Could you check a few things on this model? Use its own coordinates, in mm. A direction names the side the tool comes from. Coordinates: 2 decimals unless noted, no trailing zeros. Write each loop counter-clockwise with the first axis right and the second up, starting at its lowest first coordinate (ties: lowest second). Pieces come first, ordered by that corner, then holes.
```python
from build123d import *

# Parameters (mm, degrees)
BOSS_EXTRUDE1_REACH        = 91.067
BOSS_EXTRUDE1_START_RADIUS = 14.5
BOSS_EXTRUDE1_END_RADIUS   = 14.5
SKETCH5_W                  = 8
SKETCH5_H                  = 10
CUT_EXTRUDE1_START         = -10
CUT_EXTRUDE1_DEPTH         = 10
SKETCH8_R                  = 1.75
CUT_EXTRUDE2_DEPTH         = 3
CUT_EXTRUDE3_START         = -3
SKETCH9_R                  = 1.75
CUT_EXTRUDE3_DEPTH         = 3
CUT_EXTRUDE5_DEPTH         = 10
CUT_EXTRUDE8_START         = -10
CUT_EXTRUDE8_DEPTH         = 10
SKETCH13_R                 = 0.6
CUT_EXTRUDE9_DEPTH         = 3


# Read off the part's stored shape, not the designer's step: Cut-Extrude1, Cut-Extrude8
with BuildPart() as part:
    # Sketch1 → Revolve1 (revolve)
    with BuildSketch(Plane.XY, mode=Mode.PRIVATE) as revolve1_sk:
        with BuildLine():
            Line((12, 0), (14.5, 0))
            Line((14.5, 0), (14.5, 80))
            ThreePointArc((14.5, 80), (13.849763488, 82.244753612), (12.100400466, 83.794416583))
            Line((12.100400466, 83.794416583), (8.5, 83.794416583))
            Line((8.5, 83.794416583), (8.5, 80))
            Line((8.5, 80), (12, 80))
            Line((12, 80), (12, 0))
        make_face()
    revolve(revolve1_sk.sketch.rotate(Axis((0, 0, 0), (0, 1, 0)), 90), axis=Axis((0, 0, 0), (0, 1, 0)))

    # Boss-Extrude1: from a cylinder face, 91.067 long prism both ways, kept between that surface and its translate by the depth
    boss_extrude1_start = Plane(origin=(0, 24.058844, 0), z_dir=(0, -1, 0)) * Cylinder(BOSS_EXTRUDE1_START_RADIUS, 249.016312, mode=Mode.PRIVATE)
    boss_extrude1_end = Plane(origin=(2.8, 24.058844, 0), z_dir=(0, -1, 0)) * Cylinder(BOSS_EXTRUDE1_END_RADIUS, 249.016312, mode=Mode.PRIVATE)
    # Sketch5 → Boss-Extrude1 (add, from a surface)
    with BuildSketch(Plane(origin=(0, 0, 0), x_dir=(0, 0, -1), z_dir=(1, 0, 0)), mode=Mode.PRIVATE) as boss_extrude1_sk1:
        with Locations((-0.003167699, 5.61768818)):
            Rectangle(SKETCH5_W, SKETCH5_H)
    boss_extrude1_tool1 = extrude(boss_extrude1_sk1.sketch, amount=BOSS_EXTRUDE1_REACH, both=True, mode=Mode.PRIVATE)
    # Sketch5 → Boss-Extrude1 (add, from a surface)
    with BuildSketch(Plane(origin=(0, 0, 0), x_dir=(0, 0, -1), z_dir=(1, 0, 0)), mode=Mode.PRIVATE) as boss_extrude1_sk2:
        with Locations((0, 42.5)):
            Rectangle(SKETCH5_W, SKETCH5_H)
    boss_extrude1_tool2 = extrude(boss_extrude1_sk2.sketch, amount=BOSS_EXTRUDE1_REACH, both=True, mode=Mode.PRIVATE)
    boss_extrude1 = ((boss_extrude1_tool1 - boss_extrude1_start) & boss_extrude1_end).solids().sort_by_distance((15.337359, 5.617688, 0.003168))[0] + ((boss_extrude1_tool2 - boss_extrude1_start) & boss_extrude1_end).solids().sort_by_distance((15.337359, 5.617688, 0.003168))[0]
    add(boss_extrude1)

    # Cut-Extrude1 outline → Cut-Extrude1 (cut)
    with BuildSketch(Plane(origin=(0, 47.5, 0), x_dir=(1, 0, 0), z_dir=(0, 1, 0)).offset(CUT_EXTRUDE1_START)):
        with BuildLine():
            Line((16.737359865, 4), (13.937359865, 4))
            Line((13.937359865, 4), (16.863384202, 3.531462132))
            ThreePointArc((16.863384202, 3.531462132), (16.802331913, 3.766258222), (16.737359865, 4))
        make_face()
        with BuildLine():
            ThreePointArc((16.737359865, -4), (16.802331913, -3.766258222), (16.863384202, -3.531462132))
            Line((16.863384202, -3.531462132), (13.937359865, -4))
            Line((13.937359865, -4), (16.737359865, -4))
        make_face()
        with BuildLine():
            ThreePointArc((16.863384202, -3.531462132), (17.3, 0), (16.863384202, 3.531462132))
            Line((16.863384202, 3.531462132), (16.863384202, -3.531462132))
        make_face()
    cut_extrude1 = extrude(amount=CUT_EXTRUDE1_DEPTH, mode=Mode.SUBTRACT)

    # Mirror2: Boss-Extrude1, Cut-Extrude1 across plane
    add(boss_extrude1.mirror(Plane(origin=(0, 0, 0), x_dir=(0, 0, 1), z_dir=(1, 0, 0))))
    add(cut_extrude1.mirror(Plane(origin=(0, 0, 0), x_dir=(0, 0, 1), z_dir=(1, 0, 0))), mode=Mode.SUBTRACT)

    # Sketch8 → Cut-Extrude2 (cut)
    with BuildSketch(Plane.ZY.offset(16.863384202)):
        with Locations((0.02126458, 42.512867657)):
            Circle(SKETCH8_R)
    extrude(amount=-CUT_EXTRUDE2_DEPTH, mode=Mode.SUBTRACT)

    # Sketch9 → Cut-Extrude3 (cut)
    with BuildSketch(Plane(origin=(16.863384202, 0, 0), x_dir=(0, 0, -1), z_dir=(1, 0, 0)).offset(CUT_EXTRUDE3_START)):
        with Locations(Location((-0.02126458, 42.512867657, 0), (0, 0, 180))):
            Circle(SKETCH9_R)
    extrude(amount=CUT_EXTRUDE3_DEPTH, mode=Mode.SUBTRACT)

    # Sketch11 → Cut-Extrude5 (cut)
    with BuildSketch(Plane(origin=(0, 10.61768818, 0), x_dir=(1, 0, 0), z_dir=(0, 1, 0))):
        with BuildLine():
            Line((-13.9382686, 3.996832301), (-16.7382686, 3.996832301))
            ThreePointArc((-16.7382686, 3.996832301), (-17.299999625, -0.003295577), (-16.73645035, -4.003167699))
            Line((-16.73645035, -4.003167699), (-13.93645035, -4.003167699))
            ThreePointArc((-13.93645035, -4.003167699), (-14.499999625, -0.003295577), (-13.9382686, 3.996832301))
        make_face()
    extrude(amount=-CUT_EXTRUDE5_DEPTH, mode=Mode.SUBTRACT)

    # Cut-Extrude8 outline → Cut-Extrude8 (cut)
    with BuildSketch(Plane(origin=(0, 10.61768818, 0), x_dir=(1, 0, 0), z_dir=(0, 1, 0)).offset(CUT_EXTRUDE8_START)):
        with BuildLine():
            Line((16.7382686, 3.996832301), (13.9382686, 3.996832301))
            Line((13.9382686, 3.996832301), (17.052533954, 2.667447447))
            ThreePointArc((17.052533954, 2.667447447), (16.91106492, 3.335842745), (16.7382686, 3.996832301))
        make_face()
        with BuildLine():
            ThreePointArc((16.73645035, -4.003167699), (16.910306381, -3.339049838), (17.052533954, -2.667447447))
            Line((17.052533954, -2.667447447), (13.93645035, -4.003167699))
            Line((13.93645035, -4.003167699), (16.73645035, -4.003167699))
        make_face()
        with BuildLine():
            ThreePointArc((17.052533954, -2.667447447), (17.3, 0), (17.052533954, 2.667447447))
            Line((17.052533954, 2.667447447), (17.052533954, -2.667447447))
        make_face()
    extrude(amount=CUT_EXTRUDE8_DEPTH, mode=Mode.SUBTRACT)

    # Sketch13 → Cut-Extrude9 (cut)
    with BuildSketch(Plane(origin=(17.052533954, 0, 0), x_dir=(0, 0, -1), z_dir=(1, 0, 0))):
        with Locations((0, 4.61768818)):
            Circle(SKETCH13_R)
    extrude(amount=-CUT_EXTRUDE9_DEPTH, mode=Mode.SUBTRACT)


solid = part.part
```
1. Please list where these lines run through material, in increasing order: line 1 along X through (y, z) = (59, 0); line 2 along X through (y, z) = (7.5, -7.75); line 3 along Z through (x, y) = (0.5, 59.5).
Verdict:
line 1: x = -14.5 to -12, 12 to 14.5
line 2: x = -12.26 to -9.16, 9.16 to 12.26
line 3: z = -14.49 to -11.99, 11.99 to 14.49
2. On a 3-axis mill with a long thin cutter (end or side, diameter ignored), from which of +Z, -Z, +X, -X, +Y, -Y can I reach the whole of each face in a straight line? I mean faces 4 (the face through (13.863, 42, 0)), 5 (the face through (15.474, 5.548, -3.341)), 6 (the face through (-15.384, 44.248, -0.207)). Say none if no direction works.
Verdict:
face 4: +X
face 5: -Z, +X, -Y
face 6: -X
3. I want a section at A-A on x = 0. Please give me the cut outline in (y, z), plus the area to 3 significant figures.
Verdict:
outline: (0, -14.5) - (80, -14.5) arc R4.2 ccw to (83.79, -12.1) - (83.79, -8.5) - (80, -8.5) - (80, -12) - (0, -12) - close; (0, 12) - (80, 12) - (80, 8.5) - (83.79, 8.5) - (83.79, 12.1) arc R4.2 ccw to (80, 14.5) - (0, 14.5) - close
area: 440 mm2
4. If we mould it in two halves opening along Y, with no side actions, what happens to faces 1 (the face through (-13.863, 43, 0)), 2 (the face through (-8.2, 80, -2.8)), 3 (the face through (-16.863, 41, 2))? For each: pulls with the +Y half, pulls with the -Y half, needs draft (parallel to the pull), parting line crosses it, or undercut.
Verdict:
face 1: undercut
face 2: pulls with the -Y half
face 3: needs draft
5. I want a section at B-B on y = 61. Please give me the cut outline in (x, z).
Verdict:
outline: circle Ø29 at (0, 0); hole circle Ø24 at (0, 0)
6. For pin 1 (2.5 mm diameter, centred on x = 16, z = 0.5, fed in from +Y); pin 2 (6 mm diameter, centred on y = 66, z = 5, fed in from +X); pin 3 (6 mm diameter, centred on x = -4, z = 0, fed in from -Y); pin 4 (5 mm diameter, centred on x = 11, y = 55, fed in from +Z), each with a flat end and sliding along its axis, tell me the tip position at first contact or that it passes through.
Verdict:
pin 1: stops at y = 47.5
pin 2: stops at x = 14.36
pin 3: passes through
pin 4: stops at z = 11.75
